Source: CAD feature listing. Evaluate the final solid. Frame: model axes, mm. Face numbers are marked on the shaded views. A direction names the side the tool comes from. Round coordinates to 2 decimals unless told otherwise and drop trailing zeros. Loops run counter-clockwise (first coordinate to the right, second up) from the corner with the lowest first, then second, coordinate; pieces in that order, holes last.
(1) Section A-A, the plane z = 106.5. Return the cut outline in (x, y), plus the area to 3 significant figures.
(2) Set-up query: the marked faces 1, 2, 3, 4 and 5. Return all of +Z, -Z, +X, -X, +Y, -Y with unobstructed straight access to the full face (end or side cutting, diameter ignored); none if empty.
(3) Section B-B, the plane y = -8. Return the cut outline in (x, z).
(4) Material intervals for probe 1 along Z at (x, y) = (-42.5, -4); probe 2 along Z at (x, y) = (3, -38.1); probe 3 along Z at (x, y) = (4, -37.5), sorted ascending.
(5) Section C-C, the plane x = -14. Return the cut outline in (y, z), plus the area to 3 significant figures.
(6) Section D-D, the plane y = -21. Return the cut outline in (x, z), plus the area to 3 significant figures.
(7) First-contact query: pin 1 Ø7.5 at (x, y) = (27.5, -53.5) entering from +Z; pin 2 Ø1.5 at (x, z) = (-36.5, 98) entering from -Y; pin 3 Ø2 at (y, z) = (-61.5, 7.5) entering from -X; pin 4 Ø6 at (x, z) = (-29, 74) entering from +Y. Flat tips, straight axial feed; report the tip coordinate or a pass-through.
(8) Mould query, pull axis Z, two halves, no side actions, for the marked faces 6, 7, 8 and 9. Classes: pulls with the +Z half, pulls with the -Z half, needs draft (parallel to the pull), parting line crosses it, or undercut.
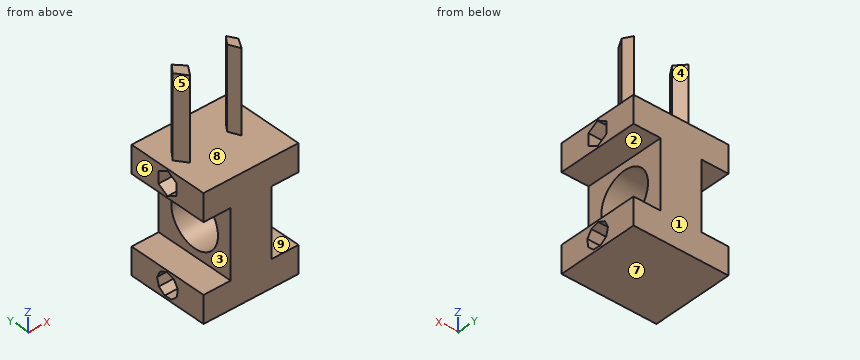
```python
from build123d import *

# Parameters (mm, degrees)
F1_DEPTH  = 76.2
F2_R      = 24.709067
F3_DEPTH  = 63.501
F5_DEPTH  = 88.901
F7_DEPTH  = 88.901
F10_DEPTH = 76.2


with BuildPart() as f1:
    # F0 (on Front) → F1 (new body)
    with BuildSketch(Plane.XZ):
        Polygon((-46.748187, -27.325264), (-46.748187, -52.725264), (42.151813, -52.725264), (42.151813, -27.325264), (16.751813, -27.325264), (16.751813, 36.174736), (42.151813, 36.174736), (42.151813, 61.574736), (-46.748187, 61.574736), (-46.748187, 36.174736), (-21.348187, 36.174736), (-21.348187, -27.325264), align=None)
    extrude(amount=F1_DEPTH)

    # F2 (on face) → F3 (cut, through all)
    with BuildSketch(Plane.YZ.offset(16.751813)):
        with Locations((-38.1, 4.424736)):
            Circle(F2_R)
    extrude(amount=-F3_DEPTH, mode=Mode.SUBTRACT)

    # F4 (on face) → F5 (cut, through all)
    with BuildSketch(Plane.YZ.offset(42.151813)):
        Polygon((-28.475514, 43.318036), (-28.475514, 54.431435), (-38.1, 59.988135), (-47.724486, 54.431435), (-47.724486, 43.318036), (-38.1, 37.761336), align=None)
    extrude(amount=-F5_DEPTH, mode=Mode.SUBTRACT)

    # F6 (on face) → F7 (cut, through all)
    with BuildSketch(Plane.YZ.offset(42.151813)):
        Polygon((-44.617329, -31.057962), (-48.856635, -37.34517), (-48.062791, -44.886425), (-42.607247, -50.153088), (-35.042712, -50.68083), (-28.908716, -46.222715), (-27.075424, -38.864743), (-30.400653, -32.049793), (-37.328493, -28.966654), align=None)
    extrude(amount=-F7_DEPTH, mode=Mode.SUBTRACT)

    # F9 (on face) → F10 (join)
    with BuildSketch(Plane.XY.offset(61.574736)):
        Polygon((-23.453956, -33.323833), (-31.261161, -24.916075), (-37.451491, -32.963499), (-30.023094, -43.177541), align=None)
        Polygon((24.142282, -32.963499), (19.499537, -24.916075), (13.618723, -32.963499), (18.261472, -43.177541), align=None)
    extrude(amount=F10_DEPTH)


solid = f1.part
```
Output values:
1. outline: (-37.45, -32.96) - (-30.02, -43.18) - (-23.45, -33.32) - (-31.26, -24.92) - close; (13.62, -32.96) - (18.26, -43.18) - (24.14, -32.96) - (19.5, -24.92) - close
1. area: 224 mm2
2. face 1: +Z, -Z, +X, -X, +Y
2. face 2: +X, +Y, -Y
2. face 3: -X, +Y, -Y
2. face 4: +Z, +Y
2. face 5: +Z, -X, -Y
3. outline: (-46.75, -52.73) - (42.15, -52.73) - (42.15, -27.33) - (16.75, -27.33) - (16.75, 36.17) - (42.15, 36.17) - (42.15, 61.57) - (-46.75, 61.57) - (-46.75, 36.17) - (-21.35, 36.17) - (-21.35, -27.33) - (-46.75, -27.33) - close
4. probe 1: z = -52.73 to -27.33, 36.17 to 61.57
4. probe 2: z = -52.73 to -50.47, -29.19 to -20.28, 29.13 to 37.76, 59.99 to 61.57
4. probe 3: z = -52.73 to -50.51, -29.02 to -20.28, 29.13 to 38.11, 59.64 to 61.57
5. outline: (-76.2, -52.73) - (0, -52.73) - (0, 61.57) - (-76.2, 61.57) - close; hole circle Ø49.42 at (-38.1, 4.42); hole (-48.86, -37.35) - (-48.06, -44.89) - (-42.61, -50.15) - (-35.04, -50.68) - (-28.91, -46.22) - (-27.08, -38.86) - (-30.4, -32.05) - (-37.33, -28.97) - (-44.62, -31.06) - close; hole (-47.72, 43.32) - (-38.1, 37.76) - (-28.48, 43.32) - (-28.48, 54.43) - (-38.1, 59.99) - (-47.72, 54.43) - close
5. area: 6,120 mm2
6. outline: (-46.75, -52.73) - (42.15, -52.73) - (42.15, -27.33) - (16.75, -27.33) - (16.75, -13.41) - (-21.35, -13.41) - (-21.35, -27.33) - (-46.75, -27.33) - close; (-46.75, 36.17) - (-21.35, 36.17) - (-21.35, 22.26) - (16.75, 22.26) - (16.75, 36.17) - (42.15, 36.17) - (42.15, 61.57) - (-46.75, 61.57) - close
6. area: 5,580 mm2
7. pin 1: stops at z = 61.57
7. pin 2: stops at y = -35.3
7. pin 3: passes through
7. pin 4: stops at y = -24.92
8. face 6: needs draft
8. face 7: pulls with the -Z half
8. face 8: pulls with the +Z half
8. face 9: undercut
